```python
from build123d import *

# Parameters (mm, degrees)
BOSS_EXTRUDE1_DEPTH      = 10
BOSS_EXTRUDE1_DEPTH_BACK = 10
SKETCH2_R                = 8.5


with BuildPart() as part:
    # Sketch1 → Revolve1 (revolve)
    with BuildSketch(Plane.XY, mode=Mode.PRIVATE) as revolve1_sk:
        Polygon((-15, 10), (-13, 10), (-13, 8), (13, 8), (13, 10), (15, 10), (15, 12), (-15, 12), align=None)
    revolve(revolve1_sk.sketch.rotate(Axis((15, 0, 0), (-1, 0, 0)), 270), axis=Axis((15, 0, 0), (-1, 0, 0)))

    # Sketch2 → Boss-Extrude1 (add, two sides: drawn at the far end of the back side and taken through both)
    with BuildSketch(Plane(origin=(0, 0, 0), x_dir=(0, 0, -1), z_dir=(1, 0, 0)).offset(-BOSS_EXTRUDE1_DEPTH_BACK)):
        with BuildLine():
            Line((-10.129868152, -5.443874651), (-10.562419487, -5.758141591))
            ThreePointArc((-10.562419487, -5.758141591), (-9.732474442, -7.071056585), (-8.740285205, -8.266094273))
            Line((-8.740285205, -8.266094273), (-8.30773387, -7.951827333))
            ThreePointArc((-8.30773387, -7.951827333), (-3.553695435, -10.937149937), (2.047131051, -11.316326898))
            Line((2.047131051, -11.316326898), (2.212350959, -11.824821489))
            ThreePointArc((2.212350959, -11.824821489), (3.717474442, -11.441209891), (5.160626159, -10.866868806))
            Line((5.160626159, -10.866868806), (4.995406251, -10.358374215))
            ThreePointArc((4.995406251, -10.358374215), (9.303695435, -6.759530401), (11.395064721, -1.55))
            Line((11.395064721, -1.55), (11.929727574, -1.55))
            ThreePointArc((11.929727574, -1.55), (12.03, 0), (11.929727574, 1.55))
            Line((11.929727574, 1.55), (11.395064721, 1.55))
            ThreePointArc((11.395064721, 1.55), (9.303695435, 6.759530401), (4.995406251, 10.358374215))
            Line((4.995406251, 10.358374215), (5.160626159, 10.866868806))
            ThreePointArc((5.160626159, 10.866868806), (3.717474442, 11.441209891), (2.212350959, 11.824821489))
            Line((2.212350959, 11.824821489), (2.047131051, 11.316326898))
            ThreePointArc((2.047131051, 11.316326898), (-3.553695435, 10.937149937), (-8.30773387, 7.951827333))
            Line((-8.30773387, 7.951827333), (-8.740285205, 8.266094273))
            ThreePointArc((-8.740285205, 8.266094273), (-9.732474442, 7.071056585), (-10.562419487, 5.758141591))
            Line((-10.562419487, 5.758141591), (-10.129868152, 5.443874651))
            ThreePointArc((-10.129868152, 5.443874651), (-11.5, 0), (-10.129868152, -5.443874651))
        make_face()
        Circle(SKETCH2_R, mode=Mode.SUBTRACT)
    extrude(amount=BOSS_EXTRUDE1_DEPTH + BOSS_EXTRUDE1_DEPTH_BACK)


solid = part.part
```
The model under review builds one solid part; all positions refer to its coordinate system, in mm. A direction names the side the tool comes from. Round coordinates to 2 decimals unless told otherwise and drop trailing zeros. Order: outer loops, then holes, each group sorted by start corner. A loop starts at its lowest first (then second) coordinate and runs counter-clockwise, first axis right, second up. Notation, with made-up numbers: M 65,80 L 117,80 A22 ccw 117,101 Z; hole C 8.5,87.5 d6. An arc over 180 degrees is marked long. Use a Markdown table: item, result.
1) Insertion check: pin 1 (12 mm diameter, centred on x = -11, y = 5.5, fed in from +Z); pin 2 (1.5 mm diameter, centred on y = -5, z = -6, fed in from +X); pin 3 (1 mm diameter, centred on x = -7.5, y = -7, fed in from +Z); pin 4 (2 mm diameter, centred on x = -3.5, y = -3, fed in from +Z). Each pin has a flat end and moves straight along its axis. Give the tip position at first contact, or say it passes through.
Report:
| item | result |
|---|---|
| pin 1 | z = 12 |
| pin 2 | x = 13 |
| pin 3 | z = 10.12 |
| pin 4 | z = 11.83 |
2) Tool access review of faces 1 (the face through (-0.14, -7.05, 9.75)), 2 (the face through (14.01, -9.76, -2.17)), 3 (the face through (-13.99, -9.76, -2.17)): name each direction out of +Z, -Z, +X, -X, +Y, -Y from which nothing blocks a thin tool from reaching the whole face with its end or side.
Report:
| item | result |
|---|---|
| face 1 | +Z, +X, -X, -Y |
| face 2 | +X |
| face 3 | -X |
3) Wall thickness on line 1 along Y through (x, z) = (13.7, 0); line 2 along X through (y, z) = (4.75, 6.5); line 3 along Y through (x, z) = (10.5, 6.5): over which ranges is each line inside the solid? List them lowest first. Write a range as [from, to].
Report:
| item | result |
|---|---|
| line 1 | [-12, -10], [10, 12] |
| line 2 | [-13, 13] |
| line 3 | [-10.09, -4.66], [4.66, 10.09] |
4) Consider section A-A (z = 0). Write out the cut boundary in (x, y), then the cut area to 3 significant figures.
Report:
| item | result |
|---|---|
| outline | M -15,-12 L 15,-12 L 15,-10 L 13,-10 L 13,-8 L -13,-8 L -13,-10 L -15,-10 Z; M -15,10 L -13,10 L -13,8 L 13,8 L 13,10 L 15,10 L 15,12 L -15,12 Z |
| area | 224 mm^2 |
5) Consider section D-D (z = -6.25). Write out the cut boundary in (x, y).
Report:
| item | result |
|---|---|
| outline | M -15,-10.24 L 15,-10.24 L 15,-7.81 L 13,-7.81 L 13,-4.99 L -13,-4.99 L -13,-7.81 L -15,-7.81 Z; M -15,7.81 L -13,7.81 L -13,4.99 L 13,4.99 L 13,7.81 L 15,7.81 L 15,10.24 L -15,10.24 Z |
6) Draft analysis for pull direction Z (two halves, no side actions). For faces 4 (the face through (-13, 8.2, 0)), 5 (the face through (-15, 9, -5)), 6 (the face through (-0.14, 7.09, 9.72)), state which applies: released by +Z, released by -Z, zero draft, split by the parting line, or undercut.
Report:
| item | result |
|---|---|
| face 4 | undercut |
| face 5 | zero draft |
| face 6 | released by +Z |
